The model under review builds one solid part; all positions refer to its coordinate system, in mm. A direction names the side the tool comes from. Coordinates: 2 decimals unless noted, no trailing zeros. Loops run counter-clockwise (first coordinate to the right, second up) from the corner with the lowest first, then second, coordinate; pieces in that order, holes last. Notation, with made-up numbers: M 87,15 L 136,15 A19 cw 136,20 Z; hole C 85.5,17 d6. An arc over 180 degrees is marked long. One line per item, written item: value.
```python
from build123d import *

# Parameters (mm, degrees)
ESQUISSE1_R        = 7.5
BOSS_EXTRU_1_DEPTH = 5.5
ESQUISSE2_R        = 3
BOSS_EXTRU_2_DEPTH = 0.5
ESQUISSE3_R        = 0.75
BOSS_EXTRU_3_DEPTH = 4.5
ESQUISSE4_R        = 2
BOSS_EXTRU_4_DEPTH = 1.4
BOSS_EXTRU_5_START = 4
ESQUISSE5_R        = 0.75
BOSS_EXTRU_5_DEPTH = 4


with BuildPart() as part:
    # Esquisse1 → Boss.-Extru.1 (new body)
    with BuildSketch(Plane.XY):
        Circle(ESQUISSE1_R)
    extrude(amount=BOSS_EXTRU_1_DEPTH)

    # Esquisse2 → Boss.-Extru.2 (add)
    with BuildSketch(Plane.XY.offset(5.5)):
        Circle(ESQUISSE2_R)
    extrude(amount=BOSS_EXTRU_2_DEPTH)

    # Esquisse3 → Boss.-Extru.3 (add)
    with BuildSketch(Plane.XY.offset(6)):
        Circle(ESQUISSE3_R)
    extrude(amount=BOSS_EXTRU_3_DEPTH)

    # Esquisse4 → Boss.-Extru.4 (add)
    with BuildSketch(Plane(origin=(0, 0, 0), x_dir=(-1, 0, 0), z_dir=(0, 0, -1))):
        with Locations(Location((0, 0, 0), (0, 0, 180))):
            Circle(ESQUISSE4_R)
    extrude(amount=BOSS_EXTRU_4_DEPTH)

    # Esquisse5 → Boss.-Extru.5 (add)
    with BuildSketch(Plane(origin=(0, 0, 0), x_dir=(-1, 0, 0), z_dir=(0, 0, -1)).offset(BOSS_EXTRU_5_START)):
        with Locations(Location((0, 0, 0), (0, 0, 180))):
            Circle(ESQUISSE5_R)
    extrude(amount=-BOSS_EXTRU_5_DEPTH)


solid = part.part
```
(1) Add section D-D on x = -1.5. State the section outline as (y, z) points.
Checks:
outline: M -7.35,0 L -1.32,0 L -1.32,-1.4 L 1.32,-1.4 L 1.32,0 L 7.35,0 L 7.35,5.5 L 2.6,5.5 L 2.6,6 L -2.6,6 L -2.6,5.5 L -7.35,5.5 Z
(2) Add section A-A on x = 0. State the section outline as (y, z) points.
Checks:
outline: M -7.5,0 L -2,0 L -2,-1.4 L -0.75,-1.4 L -0.75,-4 L 0.75,-4 L 0.75,-1.4 L 2,-1.4 L 2,0 L 7.5,0 L 7.5,5.5 L 3,5.5 L 3,6 L 0.75,6 L 0.75,10.5 L -0.75,10.5 L -0.75,6 L -3,6 L -3,5.5 L -7.5,5.5 Z
(3) Tool access review of faces 1 (the face through (1, 0, -1.4)), 2 (the face through (-3, 0.1, 5.7)), 3 (the face through (0, 0, 10.5)): name each direction out of +Z, -Z, +X, -X, +Y, -Y from which nothing blocks a thin tool from reaching the whole face with its end or side.
Checks:
face 1: -Z
face 2: +Z
face 3: +Z, +X, -X, +Y, -Y
(4) Add section C-C on z = 2.75. State the section outline as (x, y) points.
Checks:
outline: C 0,0 d15
(5) Insertion check: pin 1 Ø6.5 at (x, y) = (-1, 1.5) entering from +Z; pin 2 Ø2 at (y, z) = (4.5, 3) entering from -X; pin 3 Ø3 at (y, z) = (2.5, 3.5) entering from +X; pin 4 Ø4 at (x, y) = (-3.5, 3) entering from +Z. Each pin has a flat end and moves straight along its axis. Give the tip position at first contact, or say it passes through.
Checks:
pin 1: z = 10.5
pin 2: x = -6.63
pin 3: x = 7.43
pin 4: z = 6
(6) To check wall thickness, follow L1, parallel to Z at x = 0.25, y = -5.5; L2, parallel to Z at x = -1, y = -2; L3, parallel to Y at x = -1.5, z = -0.75. State the ranges of each line that lie inside material, in increasing order. Write a range as [from, to].
Checks:
L1: [0, 5.5]
L2: [0, 6]
L3: [-1.32, 1.32]
